Source: CAD feature listing. Evaluate the final solid. Frame: model axes, mm. Face numbers are marked on the shaded views. A direction names the side the tool comes from. Coordinates: 2 decimals unless noted, no trailing zeros.
Item 1: Contact query for flat-ended pins moving along their axis: P1, Ø3, axis at y = -134.5, z = -16, coming from the +X side; P2, Ø3, axis at y = -102.5, z = -51.5, coming from the -X side; P3, Ø6, axis at x = -116, z = -40.5, coming from the +Y side. Output: stop coordinate, or through.
Item 2: Ray query, line 1 (X direction, y = -96, z = -59); line 2 (X direction, y = -90, z = -65); line 3 (X direction, y = -145, z = -12.5). Return the intervals inside material, ascending.
Item 3: Mould query, pull axis X, two halves, no side actions, for the marked faces 4, 5 and 6. Classes: released by +X, released by -X, zero draft, split by the parting line, or undercut.
Item 4: Reachability of the marked faces 1, 2 and 3 from +Z, -Z, +X, -X, +Y, -Y: full face, straight path, thin tool, end or side. Return the list, or none.
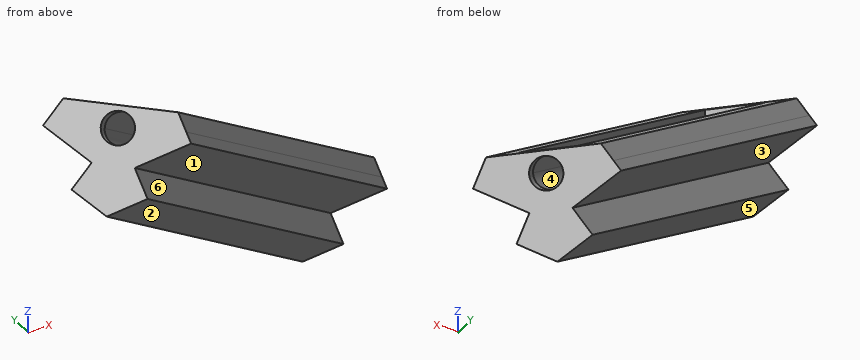
from build123d import *

# Parameters (mm, degrees)
STOCK_PFRD_START               = -164.049705188
STOCK_PFRD_JOINER_BASE_1_DEPTH = 99.013547962
BOSS_EXTRUDE1_DEPTH            = 99.013547962
CUT_EXTRUDE1_DEPTH             = 193.899706011
CUT_EXTRUDE1_DEPTH_BACK        = 193.899706011
SKETCH2_R                      = 1.55
CUT_EXTRUDE2_START             = -2
SKETCH2_3_R                    = 1.55
CUT_EXTRUDE2_DEPTH             = 95.013547962


# Read off the part's stored shape, not the designer's step: Stock-PFRD - Joiner Base-1
with BuildPart() as part:
    # Stock-PFRD - Joiner Base-1 outline → Stock-PFRD - Joiner Base-1 (new body)
    with BuildSketch(Plane(origin=(0, 0, 0), x_dir=(0.8164965809277251, -0.4082482904638628, 0.4082482904638649), z_dir=(0.5773502691896268, 0.5773502691896238, -0.5773502691896268)).offset(STOCK_PFRD_START)):
        Polygon((-62.189823503, 111.644137252), (-62.189823503, 114.644137252), (-66.189823503, 114.644137252), (-68.189823503, 111.180035637), (-65.591747292, 109.680035637), (-68.354247292, 104.895245281), (-67.382105967, 104.333979225), (-63.809678479, 110.521605141), (-56.664823503, 110.521605141), (-56.664823503, 111.644137252), align=None)
    extrude(amount=STOCK_PFRD_JOINER_BASE_1_DEPTH)

    # Sketch1 → Boss-Extrude1 (add)
    with BuildSketch(Plane(origin=(-37.548642882, -37.548642882, 37.548642882), x_dir=(-0.4082482904638644, -0.40824829046386246, -0.8164965809277256), z_dir=(0.5773502691896268, 0.5773502691896242, -0.5773502691896264))):
        Polygon((124.046929471, 6.187625915), (122.393930478, 5.233266502), (122.393930478, -5.233266502), (124.046929471, -6.187625915), (126.031643718, -2.75), (127.619356958, 0), (126.031643718, 2.75), align=None)
    extrude(amount=-BOSS_EXTRUDE1_DEPTH)

    # Sketch2 → Cut-Extrude1 (cut, two sides: drawn at the far end of the back side and taken through both)
    with BuildSketch(Plane(origin=(-37.548642882, -37.548642882, 37.548642882), x_dir=(-0.4082482904638644, -0.40824829046386246, -0.8164965809277256), z_dir=(0.5773502691896268, 0.5773502691896242, -0.5773502691896264)).offset(-CUT_EXTRUDE1_DEPTH_BACK)):
        with Locations(Location((124.443930478, 0, 0), (0, 0, 30))):
            Circle(SKETCH2_R)
    extrude(amount=CUT_EXTRUDE1_DEPTH + CUT_EXTRUDE1_DEPTH_BACK, mode=Mode.SUBTRACT)

    # Sketch2<3> → Cut-Extrude2 (cut)
    with BuildSketch(Plane(origin=(-37.548642882, -37.548642882, 37.548642882), x_dir=(-0.4082482904638644, -0.40824829046386246, -0.8164965809277256), z_dir=(0.5773502691896268, 0.5773502691896242, -0.5773502691896264)).offset(CUT_EXTRUDE2_START)):
        with BuildLine():
            Line((122.393930478, 2.799999988), (124.443930478, 2.799999988))
            ThreePointArc((124.443930478, 2.799999988), (127.243930466, 0), (124.443930478, -2.799999988))
            Line((124.443930478, -2.799999988), (122.393930478, -2.799999988))
            ThreePointArc((122.393930478, -2.799999988), (119.59393049, 0), (122.393930478, 2.799999988))
        make_face()
        with Locations(Location((124.443930478, 0, 0), (0, 0, 30))):
            Circle(SKETCH2_3_R, mode=Mode.SUBTRACT)
    extrude(amount=-CUT_EXTRUDE2_DEPTH, mode=Mode.SUBTRACT)


solid = part.part
Answer list:
1. P1: stops at x = -129.95
1. P2: stops at x = -107.89
1. P3: stops at y = -105.03
2. line 1: x = -98.89 to -97.3, -92.11 to -87.9
2. line 2: x = -92.89 to -91.3, -91.11 to -87.65
2. line 3: x = -149.63 to -135.65
3. face 4: undercut
3. face 5: released by -X
3. face 6: released by +X
4. face 1: +X, -Y
4. face 2: -Z, +X, -X, -Y
4. face 3: -X, +Y
